Here's how the part is built. I have some questions about the finished solid (model axes, mm). A direction names the side the tool comes from. Coordinates: 2 decimals unless noted, no trailing zeros. Write each loop counter-clockwise with the first axis right and the second up, starting at its lowest first coordinate (ties: lowest second). Pieces come first, ordered by that corner, then holes. Notation, with made-up numbers: (-31, -17) -> (-11, -17) arc R24 cw to (-11, 21) -> close; hole circle Ø7 at (18, 52.25). An arc over 180 degrees is marked (long way). Use a Markdown table: item, result. Add a question column.
```python
from build123d import *

# Parameters (mm, degrees)
ESQUISSE1_R                  = 6
ESQUISSE1_R_2                = 2.3
BOSS_EXTRU_1_DEPTH           = 4
ENL_V_MAT_EXTRU_1_DEPTH      = 4
ENL_V_MAT_EXTRU_2_DEPTH      = 10
ENL_V_MAT_EXTRU_2_DEPTH_BACK = 10
ESQUISSE3_R                  = 6.951264174
ESQUISSE3_R_2                = 5.333890826


with BuildPart() as part:
    # Esquisse1 → Boss.-Extru.1 (new body)
    with BuildSketch(Plane(origin=(0, 0, 0), x_dir=(1, 0, 0), z_dir=(0, 1, 0))):
        with Locations(Location((0, 0, 0), (0, 0, 270))):
            Circle(ESQUISSE1_R)
        with Locations(Location((0, 0, 0), (0, 0, 270))):
            Circle(ESQUISSE1_R_2, mode=Mode.SUBTRACT)
    extrude(amount=BOSS_EXTRU_1_DEPTH)

    # Esquisse2 → Enl_v. mat.-Extru.1 (cut)
    with BuildSketch(Plane(origin=(0, 4, 0), x_dir=(1, 0, 0), z_dir=(0, 1, 0))):
        Polygon((0.37038816, 5.988556805), (0.227331291, 4.029155081), (1.435903549, 3.678279264), (2.408685878, 5.495291834), (1.792659416, 6.071810959), align=None)
        Polygon((3.315043958, 5.001048246), (2.211452214, 3.375685011), (3.082668583, 2.467531511), (4.833629077, 3.55471939), (4.588394074, 4.36201283), align=None)
        Polygon((5.371436405, 2.673512847), (3.603016302, 1.817702868), (3.90343506, 0.595610681), (5.963405269, 0.661662757), (6.154672246, 1.483416885), align=None)
        Polygon((5.988556805, -0.37038816), (4.029155081, -0.227331291), (3.678279264, -1.435903549), (5.495291834, -2.408685878), (6.071810959, -1.792659416), align=None)
        Polygon((5.001048246, -3.315043958), (3.375685011, -2.211452214), (2.467531511, -3.082668583), (3.55471939, -4.833629077), (4.36201283, -4.588394074), align=None)
        Polygon((2.673512847, -5.371436405), (1.817702868, -3.603016302), (0.595610681, -3.90343506), (0.661662757, -5.963405269), (1.483416885, -6.154672246), align=None)
        Polygon((-0.37038816, -5.988556805), (-0.227331291, -4.029155081), (-1.435903549, -3.678279264), (-2.408685878, -5.495291834), (-1.792659416, -6.071810959), align=None)
        Polygon((-3.315043958, -5.001048246), (-2.211452214, -3.375685011), (-3.082668583, -2.467531511), (-4.833629077, -3.55471939), (-4.588394074, -4.36201283), align=None)
        Polygon((-5.371436405, -2.673512847), (-3.603016302, -1.817702868), (-3.90343506, -0.595610681), (-5.963405269, -0.661662757), (-6.154672246, -1.483416885), align=None)
        Polygon((-5.988556805, 0.37038816), (-4.029155081, 0.227331291), (-3.678279264, 1.435903549), (-5.495291834, 2.408685878), (-6.071810959, 1.792659416), align=None)
        Polygon((-5.001048246, 3.315043958), (-3.375685011, 2.211452214), (-2.467531511, 3.082668583), (-3.55471939, 4.833629077), (-4.36201283, 4.588394074), align=None)
        Polygon((-2.673512847, 5.371436405), (-1.817702868, 3.603016302), (-0.595610681, 3.90343506), (-0.661662757, 5.963405269), (-1.483416885, 6.154672246), align=None)
    extrude(amount=-ENL_V_MAT_EXTRU_1_DEPTH, mode=Mode.SUBTRACT)

    # Esquisse3 → Enl_v. mat.-Extru.2 (cut, two sides: drawn at the far end of the back side and taken through both)
    with BuildSketch(Plane(origin=(0, 4, 0), x_dir=(1, 0, 0), z_dir=(0, 1, 0)).offset(-ENL_V_MAT_EXTRU_2_DEPTH_BACK)):
        Circle(ESQUISSE3_R)
        Circle(ESQUISSE3_R_2, mode=Mode.SUBTRACT)
    extrude(amount=ENL_V_MAT_EXTRU_2_DEPTH + ENL_V_MAT_EXTRU_2_DEPTH_BACK, mode=Mode.SUBTRACT)


solid = part.part
```
Q1. Which directions (+Z, -Z, +X, -X, +Y, -Y) give clear straight access to the entire face, cutting with the end or side of a thin tool? Please do faces 5 (the flat face through (1.76, 2.03, -4.28)), 6 (the flat face through (4.196, 2.028, -2.104)), 7 (the flat face through (-2.93, 2.03, -2.64)), 8 (the cylindrical face through (-4.54, 1.97, 2.8)), 9 (the flat face through (-2.83, 2.03, -3.67)).
Q2. Thinking about a two-plate mould opening in X: for faces 1 (the cylindrical face through (-5.33, 1.97, 0.15)), 2 (the flat face through (-4.686, 2.028, -0.275)), 3 (the flat face through (3.92, 2.03, 2.58)), 4 (the cylindrical face through (2.8, 1.97, 4.54)), which applies, released by +X, released by -X, zero draft, split by the parting line, or undercut?
Q3. Suppose I cut it at B-B, the plane x = 0. Write out the boundary of the cut face in (y, z).
Q4. Please list where these lines run through material, in increasing order: line 1 (Z direction, x = -4.5, y = 1.65); line 2 (X direction, y = 2, z = 0); line 3 (X direction, y = 2.9, z = -4.5).
Q5. Suppose I cut it at A-A, the plane z = 0. Write out the boundary of the cut face in (x, y).
Q6. Will these pins go through, and if not, where does the flat tip stop? pin 1 (6 mm diameter, centred on x = 0.5, z = -1, fed in from -Y); pin 2 (1.5 mm diameter, centred on y = 1.5, z = -3.5, fed in from +X); pin 3 (2 mm diameter, centred on x = 3.5, y = 1, fed in from +Z).
Answer key:
| question | item | result |
|---|---|---|
| 1 | face 5 | -Z, +Y, -Y |
| 1 | face 6 | +X, +Y, -Y |
| 1 | face 7 | +Y, -Y |
| 1 | face 8 | +Z, -X, +Y, -Y |
| 1 | face 9 | -X, +Y, -Y |
| 2 | face 1 | released by -X |
| 2 | face 2 | undercut |
| 2 | face 3 | undercut |
| 2 | face 4 | released by +X |
| 3 | outline | (0, -5.33) -> (4, -5.33) -> (4, -2.3) -> (0, -2.3) -> close; (0, 2.3) -> (4, 2.3) -> (4, 5.33) -> (0, 5.33) -> close |
| 4 | line 1 | z = -2.86 to -1.88, -0.26 to 0.61, 2.25 to 2.86 |
| 4 | line 2 | x = -5.33 to -2.3, 2.3 to 5.33 |
| 4 | line 3 | x = -2.86 to -2.25, -0.61 to 0.26, 1.88 to 2.86 |
| 5 | outline | (-5.33, 0) -> (-2.3, 0) -> (-2.3, 4) -> (-5.33, 4) -> close; (2.3, 0) -> (5.33, 0) -> (5.33, 4) -> (2.3, 4) -> close |
| 6 | pin 1 | stops at y = 0 |
| 6 | pin 2 | stops at x = 4.57 |
| 6 | pin 3 | stops at z = 4.71 |
